```python
from build123d import *

# Parameters (mm, degrees)
SKETCH1_W                    = 152.4
SKETCH1_H                    = 25.4
BOSS_EXTRUDE1_DEPTH          = 5.08
F_12_5_12_5_DIAMETER_HOLE1_D = 12.5
FILLET3_R                    = 12.7


with BuildPart() as part:
    # Sketch1 → Boss-Extrude1 (new body)
    with BuildSketch(Plane.XY):
        Rectangle(SKETCH1_W, SKETCH1_H)
    extrude(amount=BOSS_EXTRUDE1_DEPTH)

    # Ø12.5 (12.5) Diameter Hole1 (through all)
    with Locations(Plane.XY.offset(5.08)):
        with Locations((-63.5, 0), (63.5, 0)):
            Hole(F_12_5_12_5_DIAMETER_HOLE1_D / 2)

    # Fillet3
    fillet3_edges = [part.edges().sort_by_distance(p)[0] for p in [
        (-76.2, 12.7, 2.54),
        (-76.2, -12.7, 2.54),
        (76.2, -12.7, 2.54),
        (76.2, 12.7, 2.54),
    ]]
    fillet(fillet3_edges, radius=FILLET3_R - 0.0001)  # a hair under: the kernel refuses the full size


solid = part.part
```
The listing builds one solid part. Answer for the finished solid, in the listing's coordinates (mm). Give positions to 0.01 mm unless a question says otherwise; leave off trailing zeros. Order: outer loops, then holes, each group sorted by start corner. A loop starts at its lowest first (then second) coordinate and runs counter-clockwise, first axis right, second up.
1) Determine the mould class of faces 1 (the face through (-1, 12.7, 3)), 2 (the face through (72.38, -9.08, 2.58)), 3 (the face through (57.54, 1.88, 2.5)) for opening direction X: pulls with the +X half, pulls with the -X half, needs draft (parallel to the pull), parting line crosses it, or undercut.
Reported:
face 1: needs draft
face 2: pulls with the +X half
face 3: undercut
2) Find section D-D on y = -8.25. Write down the section's boundary in (x, z), then the cut area to 3 significant figures.
Reported:
outline: (-73.16, 0) - (73.16, 0) - (73.16, 5.08) - (-73.16, 5.08) - close
area: 743 mm2
3) Given P1, Ø3, axis at y = 5.5, z = 3.5, coming from the -X side; P2, Ø3, axis at x = -60, y = -4, coming from the +Z side, each flat-ended and moving along its own axis, determine where each tip first touches the part or whether it passes through.
Reported:
P1: stops at x = -75.55
P2: stops at z = 5.08
4) Find section C-C on x = 66. Write down the section's boundary in (y, z), then the cut area to 3 significant figures.
Reported:
outline: (-12.45, 0) - (-5.73, 0) - (-5.73, 5.08) - (-12.45, 5.08) - close; (5.73, 0) - (12.45, 0) - (12.45, 5.08) - (5.73, 5.08) - close
area: 68.3 mm2
5) Consider line 1 along X through (y, z) = (1.25, 0.35); line 2 along X through (y, z) = (0.75, 2.75); line 3 along Y through (x, z) = (63.5, 3.7). Determine where each line is inside the solid, lowest interval first.
Reported:
line 1: x = -76.14 to -69.62, -57.38 to 57.38, 69.62 to 76.14
line 2: x = -76.18 to -69.7, -57.3 to 57.3, 69.7 to 76.18
line 3: y = -12.7 to -6.25, 6.25 to 12.7
6) Find section A-A on y = 2. Write down the section's boundary in (x, z), then the cut area to 3 significant figures.
Reported:
outline: (-76.04, 0) - (-69.42, 0) - (-69.42, 5.08) - (-76.04, 5.08) - close; (-57.58, 0) - (57.58, 0) - (57.58, 5.08) - (-57.58, 5.08) - close; (69.42, 0) - (76.04, 0) - (76.04, 5.08) - (69.42, 5.08) - close
area: 652 mm2
7) Find section B-B on z = 0.95. Give the number of separate pieces and of enclosed holes in the cut face, then the cut area to 3 significant figures.
Reported:
separate pieces: 1
enclosed holes: 2
area: 3,490 mm2
